For this review, take the finished solid that the model builds, in its own axes (mm). Face numbers are marked on the shaded views. Give positions to 0.01 mm unless a question says otherwise; leave off trailing zeros. Loops run counter-clockwise (first coordinate to the right, second up) from the corner with the lowest first, then second, coordinate; pieces in that order, holes last. Notation, with made-up numbers: (0.25, 12) - (43.25, 12) arc R23 ccw to (43.25, 47) - close; hole circle Ø1 at (42.5, -9.5). An arc over 180 degrees is marked (long way). Answer as CSV lines item,"result".
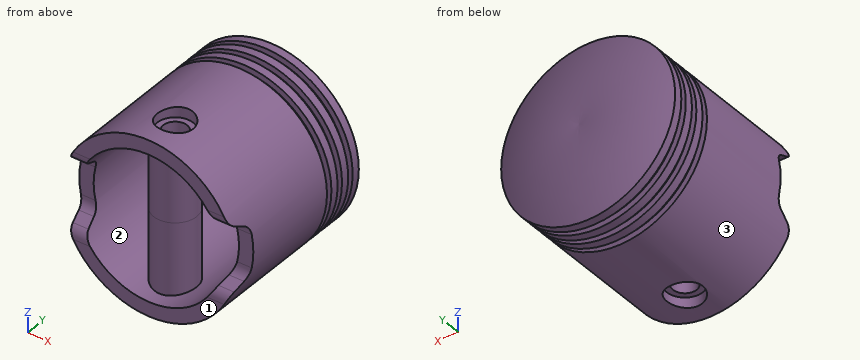
from build123d import *

# Parameters (mm, degrees)
CUT_EXTRUDE1_REACH                   = 93.307
CUT_EXTRUDE1_DIRECTION_2_REACH       = 93.307
FILLET1_R                            = 5
BOSS_EXTRUDE1_REACH                  = 93.307
BOSS_EXTRUDE1_END_RADIUS             = 30.50852022
SKETCH3_R                            = 9
BOSS_EXTRUDE1_DIRECTION_2_REACH      = 93.307
BOSS_EXTRUDE1_DIRECTION_2_END_RADIUS = 30.50852022
CUT_EXTRUDE2_REACH                   = 93.307
CUT_EXTRUDE2_END_RADIUS              = 36.50852022
SKETCH4_R                            = 5
CUT_EXTRUDE2_DIRECTION_2_REACH       = 93.307
CUT_EXTRUDE2_DIRECTION_2_END_RADIUS  = 36.50852022
SKETCH5_R                            = 7.5
CUT_EXTRUDE3_DEPTH                   = 10


with BuildPart() as part:
    # Sketch1 → Revolve1 (revolve)
    with BuildSketch(Plane.XY, mode=Mode.PRIVATE) as revolve1_sk:
        with BuildLine():
            Line((0, 65.6), (0, 70))
            Line((0, 70), (0, 75))
            ThreePointArc((0, 75), (-18.565651024, 74.469071932), (-36.50852022, 69.671288317))
            Line((-36.50852022, 69.671288317), (-36.50852022, 66.171288317))
            Line((-36.50852022, 66.171288317), (-34.00852022, 66.171288317))
            Line((-34.00852022, 66.171288317), (-34.00852022, 63.671288317))
            Line((-34.00852022, 63.671288317), (-36.50852022, 63.671288317))
            Line((-36.50852022, 63.671288317), (-36.50852022, 60.171288317))
            Line((-36.50852022, 60.171288317), (-34.00852022, 60.171288317))
            Line((-34.00852022, 60.171288317), (-34.00852022, 57.671288317))
            Line((-34.00852022, 57.671288317), (-36.50852022, 57.671288317))
            Line((-36.50852022, 57.671288317), (-36.50852022, 54.171288317))
            Line((-36.50852022, 54.171288317), (-34.00852022, 54.171288317))
            Line((-34.00852022, 54.171288317), (-34.00852022, 51.671288317))
            Line((-34.00852022, 51.671288317), (-36.50852022, 51.671288317))
            Line((-36.50852022, 51.671288317), (-36.50852022, 0))
            Line((-36.50852022, 0), (-30.50852022, 0))
            Line((-30.50852022, 0), (-30.50852022, 65.6))
            Line((-30.50852022, 65.6), (0, 65.6))
        make_face()
    revolve(revolve1_sk.sketch.rotate(Axis((0, 70, 0), (0, 1, 0)), 270), axis=Axis((0, 70, 0), (0, 1, 0)))

    # Sketch2 → Cut-Extrude1 (cut, up to next)
    with BuildSketch(Plane(origin=(0, 0, 0), x_dir=(0, 0, -1), z_dir=(1, 0, 0)), mode=Mode.PRIVATE) as cut_extrude1_sk1:
        Polygon((-15, 0), (-10, 10), (10, 10), (15, 0), align=None)
    cut_extrude1_tool1 = extrude(cut_extrude1_sk1.sketch, amount=-CUT_EXTRUDE1_REACH, mode=Mode.PRIVATE) & part.part
    add(cut_extrude1_tool1.solids().sort_by_distance((0, 4.666667, 0))[0], mode=Mode.SUBTRACT)

    # Sketch2 → Cut-Extrude1 direction 2 (cut, up to next)
    with BuildSketch(Plane(origin=(0, 0, 0), x_dir=(0, 0, -1), z_dir=(1, 0, 0)), mode=Mode.PRIVATE) as cut_extrude1_direction_2_sk1:
        Polygon((-15, 0), (-10, 10), (10, 10), (15, 0), align=None)
    cut_extrude1_direction_2_tool1 = extrude(cut_extrude1_direction_2_sk1.sketch, amount=CUT_EXTRUDE1_DIRECTION_2_REACH, mode=Mode.PRIVATE) & part.part
    add(cut_extrude1_direction_2_tool1.solids().sort_by_distance((0, 4.666667, 0))[0], mode=Mode.SUBTRACT)

    # Fillet1
    fillet1_edges = [part.edges().sort_by_distance(p)[0] for p in [
        (31.967677706, 10, -10),
        (-31.967677706, 10, -10),
        (29.92552018, 0, -15),
        (-29.92552018, 0, -15),
        (31.967677706, 10, 10),
        (-31.967677706, 10, 10),
        (-29.92552018, 0, 15),
        (29.92552018, 0, 15),
    ]]
    fillet(fillet1_edges, radius=FILLET1_R)

    # Boss-Extrude1: up to this cylinder (the profile starts inside it)
    boss_extrude1_end = Plane(origin=(0, 15, 0), z_dir=(0, -1, 0)) * Cylinder(BOSS_EXTRUDE1_END_RADIUS, 248.631040439, mode=Mode.PRIVATE)
    # Sketch3 → Boss-Extrude1 (add, up to the surface)
    with BuildSketch(Plane.XY, mode=Mode.PRIVATE) as boss_extrude1_sk1:
        with Locations((0, 15)):
            Circle(SKETCH3_R)
    boss_extrude1_tool1 = extrude(boss_extrude1_sk1.sketch, amount=BOSS_EXTRUDE1_REACH, mode=Mode.PRIVATE) & boss_extrude1_end
    add(boss_extrude1_tool1.solids().sort_by_distance((0, 15, 0))[0])

    # Boss-Extrude1 direction 2: up to this cylinder (the profile starts inside it)
    boss_extrude1_direction_2_end = Plane(origin=(0, 15, 0), z_dir=(0, -1, 0)) * Cylinder(BOSS_EXTRUDE1_DIRECTION_2_END_RADIUS, 248.631040439, mode=Mode.PRIVATE)
    # Sketch3 → Boss-Extrude1 direction 2 (add, up to the surface)
    with BuildSketch(Plane.XY, mode=Mode.PRIVATE) as boss_extrude1_direction_2_sk1:
        with Locations((0, 15)):
            Circle(SKETCH3_R)
    boss_extrude1_direction_2_tool1 = extrude(boss_extrude1_direction_2_sk1.sketch, amount=-BOSS_EXTRUDE1_DIRECTION_2_REACH, mode=Mode.PRIVATE) & boss_extrude1_direction_2_end
    add(boss_extrude1_direction_2_tool1.solids().sort_by_distance((0, 15, 0))[0])

    # Cut-Extrude2: up to this cylinder (the profile starts inside it)
    cut_extrude2_end = Plane(origin=(0, 15, 0), z_dir=(0, -1, 0)) * Cylinder(CUT_EXTRUDE2_END_RADIUS, 260.631040439, mode=Mode.PRIVATE)
    # Sketch4 → Cut-Extrude2 (cut, up to the surface)
    with BuildSketch(Plane.XY, mode=Mode.PRIVATE) as cut_extrude2_sk1:
        with Locations(Location((0, 15, 0), (0, 0, 180))):
            Circle(SKETCH4_R)
    cut_extrude2_tool1 = extrude(cut_extrude2_sk1.sketch, amount=-CUT_EXTRUDE2_REACH, mode=Mode.PRIVATE) & cut_extrude2_end
    add(cut_extrude2_tool1.solids().sort_by_distance((0, 15, 0))[0], mode=Mode.SUBTRACT)

    # Cut-Extrude2 direction 2: up to this cylinder (the profile starts inside it)
    cut_extrude2_direction_2_end = Plane(origin=(0, 15, 0), z_dir=(0, -1, 0)) * Cylinder(CUT_EXTRUDE2_DIRECTION_2_END_RADIUS, 260.631040439, mode=Mode.PRIVATE)
    # Sketch4 → Cut-Extrude2 direction 2 (cut, up to the surface)
    with BuildSketch(Plane.XY, mode=Mode.PRIVATE) as cut_extrude2_direction_2_sk1:
        with Locations(Location((0, 15, 0), (0, 0, 180))):
            Circle(SKETCH4_R)
    cut_extrude2_direction_2_tool1 = extrude(cut_extrude2_direction_2_sk1.sketch, amount=CUT_EXTRUDE2_DIRECTION_2_REACH, mode=Mode.PRIVATE) & cut_extrude2_direction_2_end
    add(cut_extrude2_direction_2_tool1.solids().sort_by_distance((0, 15, 0))[0], mode=Mode.SUBTRACT)

    # Sketch5 → Cut-Extrude3 (cut)
    with BuildSketch(Plane.XY.offset(32)):
        with Locations(Location((0, 15, 0), (0, 0, 180))):
            Circle(SKETCH5_R)
    cut_extrude3 = extrude(amount=CUT_EXTRUDE3_DEPTH, mode=Mode.SUBTRACT)

    # Mirror1: Cut-Extrude3 across plane
    add(cut_extrude3.mirror(Plane.XY), mode=Mode.SUBTRACT)


solid = part.part
1) Draft analysis for pull direction X (two halves, no side actions). For the marked faces 1, 2 and 3, state which applies: pulls with the +X half, pulls with the -X half, needs draft (parallel to the pull), parting line crosses it, or undercut.
From the geometry:
face 1,"needs draft"
face 2,"undercut"
face 3,"parting line crosses it"
2) Consider section B-B on z = -20. Count the separate pieces of the cut face and the enclosed holes in it, and give its area (3 significant figures).
From the geometry:
separate pieces,"2"
enclosed holes,"1"
area,"1,550 mm^2"
3) Insertion check: P1, Ø8, axis at x = -1, z = -27, coming from the -Y side; P2, Ø5.5, axis at x = 32, z = -1, coming from the -Y side; P3, Ø2, axis at y = 32, z = -0.5, coming from the +X side; P4, Ø7.5, axis at x = 1.5, y = 18, coming from the -Z side. Each pin has a flat end and moves straight along its axis. Give the tip position at first contact, or say it passes through.
From the geometry:
P1,"stops at y = 0"
P2,"stops at y = 10"
P3,"stops at x = 36.51"
P4,"stops at z = -32"
4) Wall thickness on line 1 (Y direction, x = 3.5, z = 18); line 2 (Y direction, x = 1, z = 1); line 3 (X direction, y = 18.5, z = 19.5): over which ranges is each line inside the solid? List them lowest first. Write a range as from..to.
From the geometry:
line 1,"y = 6.71..11.43, 18.57..23.29, 65.6..74.5"
line 2,"y = 6.06..10.1, 19.9..23.94, 65.6..75.11"
line 3,"x = -30.86..-23.46, -8.29..-3.57, 3.57..8.29, 23.46..30.86"
5) Consider section A-A on y = 15. Write out the cut boundary in (x, z).
From the geometry:
outline,"(-7.5, -35.73) - (-7.5, -32) - (-5, -32) - (-5, 32) - (-7.5, 32) - (-7.5, 35.73) arc R36.51 ccw to start; (5, -32) - (7.5, -32) - (7.5, -35.73) arc R36.51 ccw to (7.5, 35.73) - (7.5, 32) - (5, 32) - close; hole (-9, -29.15) - (-9, 29.15) arc R30.51 ccw to start; hole (9, -29.15) arc R30.51 ccw to (9, 29.15) - close"
6) Consider section C-C on y = 48.5. Write out the cut boundary in (x, z), and give its area (3 significant figures).
From the geometry:
outline,"circle Ø73.02 at (0, 0); hole circle Ø61.02 at (0, 0)"
area,"1,260 mm^2"
